Could you check a few things on this model? Use its own coordinates, in mm. A direction names the side the tool comes from. Give positions to 0.01 mm unless a question says otherwise; leave off trailing zeros. Order: outer loops, then holes, each group sorted by start corner. A loop starts at its lowest first (then second) coordinate and runs counter-clockwise, first axis right, second up.
(1) Imagine slicing it at A-A, the plane z = 10. Write out the boundary of the cut face in (x, y).
(2) On a 3-axis mill with a long thin cutter (end or side, diameter ignored), from which of +Z, -Z, +X, -X, +Y, -Y can I reach the whole of each face in a straight line? I mean faces 4 (the flat face through (10, -17, 10)), 5 (the flat face through (18, -15, 10)). Say none if no direction works.
(3) If we mould it in two halves opening along X, with no side actions, what happens to faces 1 (the flat face through (11, -12.3, 7.6)), 2 (the flat face through (14, -5, 10)), 3 (the cylindrical face through (15.772, -16.014, 11.735))? For each: released by +X, released by -X, zero draft, split by the parting line, or undercut.
(4) Imagine slicing it at B-B, the plane x = 16. Write out the boundary of the cut face in (y, z).
(5) Imagine slicing it at D-D, the plane x = 11.5. Write out the boundary of the cut face in (y, z), then the cut area to 3 significant figures.
(6) Imagine slicing it at C-C, the plane y = -10. Write out the boundary of the cut face in (x, z).
(7) If I drill on probe 1 along Z at (x, y) = (16, -4.15); probe 2 along Y at (x, z) = (17.5, 12.5); probe 3 along Y at (x, z) = (7.5, 10), over which ranges is the centre line in solid material (lowest first)?
Autodesk Inventor part; units mm, degrees
ref_plane "YZ Plane" through (0, 0, 0) normal (1, 0, 0) x (0, 1, 0)
ref_plane "XZ Plane" through (0, 0, 0) normal (0, 1, 0) x (-1, 0, 0)
ref_plane "XY Plane" through (0, 0, 0) normal (0, 0, 1) x (1, 0, 0)
sketch "Sketch1" plane through (0, 0, 0) normal (0, 0, 1) x (1, 0, 0)
  line L0 (0, 0) -> (0, -20)
  line L1 (0, -20) -> (21, -20)
  line L2 (21, -20) -> (21, -15)
  line L3 (21, -15) -> (11, -15)
  line L4 (11, -15) -> (11, -5)
  line L5 (11, -5) -> (21, -5)
  line L6 (21, -5) -> (21, 0)
  line L7 (21, 0) -> (0, 0)
  dimension "d0" = 20
  dimension "d1" = 21
  dimension "d2" = 5
  dimension "d3" = 10
  dimension "d4" = 10
  dimension "d5" = 90
extrude "Extrusion1" add sketch "Sketch1" along normal blind 20
sketch "Sketch2" plane through (0, 0, 20) normal (0, 0, 1) x (1, 0, 0)
  point P0 (0, 0)
sketch "Sketch3" plane through (0, -20, 0) normal (-1, 0, 0) x (0, 0, 1)
  point P0 (0, 20)
sketch "Sketch4" plane through (0, -20, 0) normal (-1, 0, 0) x (0, 0, 1)
  line L0 (20, 20) -> (20, 0)
  line L1 (0, 20) -> (20, 20)
  line L2 (20, 20) -> (20, 0)
  line L3 (20, 0) -> (0, 0)
  line L4 (0, 0) -> (0, 20)
  circle A0 centre (10, 10) radius 2.75
  dimension "d8" = 5.5
  dimension "d9" = 10
  dimension "d10" = 10
extrude "Extrusion2" cut sketch "Sketch4" against normal blind 11 contours A0
sketch "Sketch5" plane through (0, 0, 0) normal (0, 1, 0) x (1, 0, 0)
  point P0 (0, 0)
sketch "Sketch6" plane through (0, 0, 0) normal (0, 1, 0) x (1, 0, 0)
  line L0 (21, 0) -> (21, -20)
  line L1 (0, 0) -> (21, 0)
  line L2 (21, 0) -> (21, -20)
  line L3 (21, -20) -> (0, -20)
  line L4 (0, -20) -> (0, 0)
extrude "Extrusion3" cut sketch "Sketch6" against normal blind 3
sketch "Sketch7" plane through (0, -20, 0) normal (0, -1, 0) x (1, 0, 0)
  line L0 (0, 0) -> (21, 0)
  line L1 (0, 20) -> (21, 20)
  line L2 (0, 0) -> (21, 0)
  line L3 (21, 0) -> (21, 20)
  line L4 (21, 20) -> (0, 20)
  line L5 (0, 20) -> (0, 0)
extrude "Extrusion4" cut sketch "Sketch7" against normal blind 3
sketch "Sketch8" plane through (0, -3, 0) normal (0, 1, 0) x (1, 0, 0)
  point P0 (0, 0)
sketch "Sketch9" plane through (0, -3, 0) normal (0, 1, 0) x (1, 0, 0)
  line L0 (0, -20) -> (21, -20)
  line L1 (0, 0) -> (21, 0)
  line L2 (21, 0) -> (21, -20)
  line L3 (21, -20) -> (0, -20)
  line L4 (0, -20) -> (0, 0)
  line L5 (0, 0) -> (21, 0)
  line L6 (0, 0) -> (11, 0)
  line L7 (11, 0) -> (11, -20)
  circle A0 centre (16, -10) radius 1.75
  dimension "d17" = 11
  dimension "d18" = 3.5
  dimension "d19" = 5
  dimension "d20" = 10
extrude "Extrusion5" cut sketch "Sketch9" against normal blind 3.5 contours A0
sketch "Sketch10" plane through (0, -17, 0) normal (0, -1, 0) x (1, 0, 0)
  line L0 (11, 20) -> (21, 20)
  line L1 (0, 0) -> (21, 0)
  line L2 (21, 0) -> (21, 20)
  line L3 (21, 20) -> (0, 20)
  line L4 (0, 20) -> (0, 0)
  line L5 (11, 0) -> (11, 20)
  line L6 (11, 20) -> (11, 0)
  circle A0 centre (16, 10) radius 1.75
  dimension "d23" = 3.5
  dimension "d24" = 5
  dimension "d25" = 10
extrude "Extrusion6" cut sketch "Sketch10" against normal blind 3.5 contours A0
properties part number "Encaixe Bandeja-Motor"
Answer block:
1. outline: (0, -17) - (14.25, -17) - (14.25, -15) - (11, -15) - (11, -12.75) - (0, -12.75) - close; (0, -7.25) - (11, -7.25) - (11, -5) - (14.25, -5) - (14.25, -3) - (0, -3) - close; (17.75, -17) - (21, -17) - (21, -15) - (17.75, -15) - close; (17.75, -5) - (21, -5) - (21, -3) - (17.75, -3) - close
2. face 4: +Z, -Z, +X, -X, -Y
2. face 5: +Z, -Z, +X
3. face 1: released by +X
3. face 2: zero draft
3. face 3: undercut
4. outline: (-17, 0) - (-15, 0) - (-15, 8.25) - (-17, 8.25) - close; (-17, 11.75) - (-15, 11.75) - (-15, 20) - (-17, 20) - close; (-5, 0) - (-3, 0) - (-3, 8.25) - (-5, 8.25) - close; (-5, 11.75) - (-3, 11.75) - (-3, 20) - (-5, 20) - close
5. outline: (-17, 0) - (-15, 0) - (-15, 20) - (-17, 20) - close; (-5, 0) - (-3, 0) - (-3, 20) - (-5, 20) - close
5. area: 80.0 mm2
6. outline: (0, 0) - (11, 0) - (11, 7.25) - (0, 7.25) - close; (0, 12.75) - (11, 12.75) - (11, 20) - (0, 20) - close
7. probe 1: z = 0 to 8.25, 11.75 to 20
7. probe 2: y = -17 to -15, -5 to -3
7. probe 3: y = -17 to -12.75, -7.25 to -3
